Read the model definition and answer for the solid it produces. Units are mm, in the model's axes. A direction names the side the tool comes from. Coordinates: 2 decimals unless noted, no trailing zeros. Order: outer loops, then holes, each group sorted by start corner. A loop starts at its lowest first (then second) coordinate and runs counter-clockwise, first axis right, second up. Notation, with made-up numbers: M 68.25,83.25 L 74.25,83.25 A23 ccw 74.25,101.25 Z; hole C 9,5 d3. An arc over 180 degrees is marked long. Use a Markdown table: item, result. Add a question column.
1) Find section A-A on y = -1. Write down the section's boundary in (x, z), plus the area to 3 significant figures.
2) For faces 1 (the face through (-10, -2, 16)), 2 (the face through (-8.5, -2, 18)), 3 (the face through (0, 1, -20)), determine the directions among +Z, -Z, +X, -X, +Y, -Y from which every point of the face is accessible in a straight line to the end or side of a thin tool.
3) The mould has two halves that part along X. Classify faces 4 (the face through (12.5, 1, 0)), 5 (the face through (-10, -2, -16)), 6 (the face through (0, 0, 0)), 7 (the face through (8.5, -2, 18)): released by +X, released by -X, zero draft, split by the parting line, or undercut.
4) Find section B-B on z = 18. Write down the section's boundary in (x, y), plus the area to 3 significant figures.
5) Find the intervals of material crossed by probe 1 along X at (y, z) = (-1.3, -18); probe 2 along X at (y, z) = (0.75, 18); probe 3 along Z at (x, y) = (10.5, -0.65), in increasing order. Write a range as [from, to].
6) Find section D-D on x = -3. Write down the section's boundary in (y, z), plus the area to 3 significant figures.
7) This flat-tipped pin is pushed along its axis until it touches: pin 1 Ø3 at (x, z) = (-2.5, -12.5) entering from -Y. Where does it stop, or does it pass through?
8) Find section C-C on x = 10.5. Write down the section's boundary in (y, z).
from build123d import *

# Parameters (mm, degrees)
SKETCH1_W           = 25
SKETCH1_H           = 40
SKETCH1_R           = 0.95
BOSS_EXTRUDE1_DEPTH = 2
BOSS_EXTRUDE2_START = 3
SKETCH2_W           = 4
SKETCH2_H           = 4
SKETCH2_R           = 0.95
BOSS_EXTRUDE2_DEPTH = 3


with BuildPart() as part:
    # Sketch1 → Boss-Extrude1 (new body)
    with BuildSketch(Plane(origin=(0, 0, 0), x_dir=(1, 0, 0), z_dir=(0, 1, 0))):
        Rectangle(SKETCH1_W, SKETCH1_H)
        with Locations(Location((-10.5, 18, 0), (0, 0, 270))):
            Circle(SKETCH1_R, mode=Mode.SUBTRACT)
        with Locations(Location((10.5, 18, 0), (0, 0, 90))):
            Circle(SKETCH1_R, mode=Mode.SUBTRACT)
        with Locations(Location((-10.5, -18, 0), (0, 0, 90))):
            Circle(SKETCH1_R, mode=Mode.SUBTRACT)
        with Locations(Location((10.5, -18, 0), (0, 0, 270))):
            Circle(SKETCH1_R, mode=Mode.SUBTRACT)
    extrude(amount=BOSS_EXTRUDE1_DEPTH)

    # Sketch2 → Boss-Extrude2 (add)
    # profile 1 of 4: a face of its own
    with BuildSketch(Plane(origin=(0, 0, 0), x_dir=(-1, 0, 0), z_dir=(0, -1, 0)).offset(BOSS_EXTRUDE2_START)):
        with Locations((-10.5, 18)):
            Rectangle(SKETCH2_W, SKETCH2_H)
        with Locations(Location((-10.5, 18, 0), (0, 0, 90))):
            Circle(SKETCH2_R, mode=Mode.SUBTRACT)
    # profile 2 of 4: a face of its own
    with BuildSketch(Plane(origin=(0, 0, 0), x_dir=(-1, 0, 0), z_dir=(0, -1, 0)).offset(BOSS_EXTRUDE2_START)):
        with Locations((10.5, 18)):
            Rectangle(SKETCH2_W, SKETCH2_H)
        with Locations(Location((10.5, 18, 0), (0, 0, 270))):
            Circle(SKETCH2_R, mode=Mode.SUBTRACT)
    # profile 3 of 4: a face of its own
    with BuildSketch(Plane(origin=(0, 0, 0), x_dir=(-1, 0, 0), z_dir=(0, -1, 0)).offset(BOSS_EXTRUDE2_START)):
        with Locations((-10.5, -18)):
            Rectangle(SKETCH2_W, SKETCH2_H)
        with Locations(Location((-10.5, -18, 0), (0, 0, 270))):
            Circle(SKETCH2_R, mode=Mode.SUBTRACT)
    # profile 4 of 4: a face of its own
    with BuildSketch(Plane(origin=(0, 0, 0), x_dir=(-1, 0, 0), z_dir=(0, -1, 0)).offset(BOSS_EXTRUDE2_START)):
        with Locations((10.5, -18)):
            Rectangle(SKETCH2_W, SKETCH2_H)
        with Locations(Location((10.5, -18, 0), (0, 0, 90))):
            Circle(SKETCH2_R, mode=Mode.SUBTRACT)
    extrude(amount=-BOSS_EXTRUDE2_DEPTH)


solid = part.part
Check result:
| question | item | result |
|---|---|---|
| 1 | outline | M -12.5,-20 L -8.5,-20 L -8.5,-16 L -12.5,-16 Z; M -12.5,16 L -8.5,16 L -8.5,20 L -12.5,20 Z; M 8.5,-20 L 12.5,-20 L 12.5,-16 L 8.5,-16 Z; M 8.5,16 L 12.5,16 L 12.5,20 L 8.5,20 Z; hole C -10.5,-18 d1.9; hole C -10.5,18 d1.9; hole C 10.5,-18 d1.9; hole C 10.5,18 d1.9 |
| 1 | area | 52.7 mm2 |
| 2 | face 1 | +X, -X, -Y |
| 2 | face 2 | +Z, -Z, -Y |
| 2 | face 3 | -Z, +X, -X, +Y, -Y |
| 3 | face 4 | released by +X |
| 3 | face 5 | zero draft |
| 3 | face 6 | undercut |
| 3 | face 7 | undercut |
| 4 | outline | M -12.5,-3 L -11.45,-3 L -11.45,2 L -12.5,2 Z; M -9.55,-3 L -8.5,-3 L -8.5,0 L 8.5,0 L 8.5,-3 L 9.55,-3 L 9.55,2 L -9.55,2 Z; M 11.45,-3 L 12.5,-3 L 12.5,2 L 11.45,2 Z |
| 4 | area | 55.0 mm2 |
| 5 | probe 1 | x = [-12.5, -11.45], [-9.55, -8.5], [8.5, 9.55], [11.45, 12.5] |
| 5 | probe 2 | x = [-12.5, -11.45], [-9.55, 9.55], [11.45, 12.5] |
| 5 | probe 3 | z = [-20, -18.95], [-17.05, -16], [16, 17.05], [18.95, 20] |
| 6 | outline | M 0,-20 L 2,-20 L 2,20 L 0,20 Z |
| 6 | area | 80.0 mm2 |
| 7 | pin 1 | stops at y = 0 |
| 8 | outline | M -3,-20 L 2,-20 L 2,-18.95 L -3,-18.95 Z; M -3,-17.05 L 2,-17.05 L 2,17.05 L -3,17.05 L -3,16 L 0,16 L 0,-16 L -3,-16 Z; M -3,18.95 L 2,18.95 L 2,20 L -3,20 Z |
